```python
from build123d import *

# Parameters (mm, degrees)
CUT_EXTRUDE1_START = 11
CUT_EXTRUDE1_DEPTH = 690.321354808


with BuildPart() as part:
    # Sketch1 → Revolve1 (revolve)
    with BuildSketch(Plane(origin=(0, 0, 0), x_dir=(0, 0, -1), z_dir=(1, 0, 0)), mode=Mode.PRIVATE) as revolve1_sk:
        Polygon((0, 15), (70, 15), (70, 12.5), (90, 12.5), (90, 15), (580, 15), (580, 12.5), (600, 12.5), (600, 15), (670, 15), (670, 12.5), (700, 12.5), (700, 0), (-30, 0), (-30, 12.5), (0, 12.5), align=None)
    revolve(revolve1_sk.sketch.rotate(Axis((0, 0, 91.723358082), (0, 0, -1)), 90), axis=Axis((0, 0, 91.723358082), (0, 0, -1)))

    # Sketch2 → Cut-Extrude1 (cut, through all)
    with BuildSketch(Plane(origin=(0, 0, 0), x_dir=(1, 0, 0), z_dir=(0, 1, 0)).offset(CUT_EXTRUDE1_START)):
        with BuildLine():
            Line((4, 646), (4, 624))
            ThreePointArc((4, 624), (0, 620), (-4, 624))
            Line((-4, 624), (-4, 646))
            ThreePointArc((-4, 646), (0, 650), (4, 646))
        make_face()
        with BuildLine():
            Line((4, 372), (4, 350))
            ThreePointArc((4, 350), (0, 346), (-4, 350))
            Line((-4, 350), (-4, 372))
            ThreePointArc((-4, 372), (0, 376), (4, 372))
        make_face()
        with BuildLine():
            Line((4, 46), (4, 24))
            ThreePointArc((4, 24), (0, 20), (-4, 24))
            Line((-4, 24), (-4, 46))
            ThreePointArc((-4, 46), (0, 50), (4, 46))
        make_face()
    extrude(amount=CUT_EXTRUDE1_DEPTH, mode=Mode.SUBTRACT)


solid = part.part
```
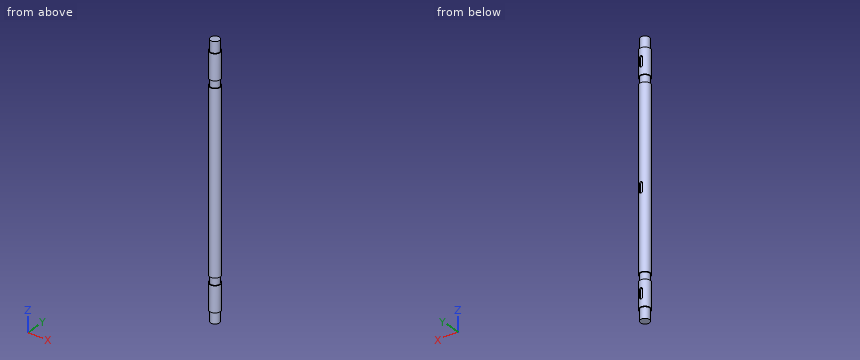
Design review of the part built by this model. Coordinates are the model's own, in mm. Round coordinates to 2 decimals unless told otherwise and drop trailing zeros. Write each loop counter-clockwise with the first axis right and the second up, starting at its lowest first coordinate (ties: lowest second). Pieces come first, ordered by that corner, then holes.
Item 1: For probe 1 along Z at (x, y) = (-4, -13); probe 2 along Y at (x, z) = (8.5, -97.5); probe 3 along Y at (x, z) = (1, -266), list the stretches that pass through material, from the lowest coordinate up.
Item 2: We need section B-B on z = -591.5. Write out the cut boundary in (x, y), and give its area (3 significant figures).
Item 3: We need section A-A on y = 0. Write out the cut boundary in (x, z), and give its area (3 significant figures).
Item 4: We need section C-C on z = -275.5. Write out the cut boundary in (x, y).
Item 5: Clearance check with flat-ended pins moving along their axes: pin 1 Ø5 at (y, z) = (10.5, -543) entering from +X; pin 2 Ø6 at (y, z) = (-5.5, -283) entering from -X; pin 3 Ø1.5 at (y, z) = (6, -256) entering from -X. State where each tip first meets the part, or that it passes through.
Returned:
1. probe 1: z = -670 to -600, -580 to -90, -70 to 0
1. probe 2: y = -12.36 to 12.36
1. probe 3: y = -14.97 to 14.97
2. outline: circle Ø25 at (0, 0)
2. area: 491 mm2
3. outline: (-15, -670) - (-12.5, -670) - (-12.5, -700) - (12.5, -700) - (12.5, -670) - (15, -670) - (15, -600) - (12.5, -600) - (12.5, -580) - (15, -580) - (15, -90) - (12.5, -90) - (12.5, -70) - (15, -70) - (15, 0) - (12.5, 0) - (12.5, 30) - (-12.5, 30) - (-12.5, 0) - (-15, 0) - (-15, -70) - (-12.5, -70) - (-12.5, -90) - (-15, -90) - (-15, -580) - (-12.5, -580) - (-12.5, -600) - (-15, -600) - close
3. area: 21,400 mm2
4. outline: circle Ø30 at (0, 0)
5. pin 1: stops at x = 12.69
5. pin 2: stops at x = -14.79
5. pin 3: stops at x = -14.05
